Read the model definition and answer for the solid it produces. Units are mm, in the model's axes. Coordinates: 2 decimals unless noted, no trailing zeros. Write each loop counter-clockwise with the first axis right and the second up, starting at its lowest first coordinate (ties: lowest second). Pieces come first, ordered by that corner, then holes.
Item 1: Each of these flat-tipped pins is pushed along its axis until it touches: P1, Ø12.5, axis at x = 12.7, y = -31.24, coming from the +Z side; P2, Ø2, axis at y = 10.5, z = 1, coming from the -X side; P3, Ø1.5, axis at x = -49, z = 2, coming from the -Y side; P4, Ø1, axis at x = 19.5, z = 3, coming from the +Y side. Where does it stop, or does it pass through?
Item 2: Section C-C (z = 1.75) is taken. State how many separate pieces and enclosed holes the cut face has, then the cut area to 3 significant figures.
Item 3: Straight lines are drawn through the part: probe 1 along X at (y, z) = (0.5, 6); probe 2 along X at (y, z) = (-27.5, 4.5); probe 3 along Y at (x, z) = (-12.7, 2.75). For each, find the intervals that lie inside material, in ascending order.
Item 4: Section A-A (x = -31.75) is taken. Give the vertices of the cut face in (y, z) (3 decimals), then the cut area to 3 significant figures.
Item 5: Section B-B (y = 26) is taken. Give the vertices of the cut face in (x, z) (3 decimals).
Item 6: Section D-D (y = -38) is taken. Give the vertices of the cut face in (x, z) (3 decimals), then the cut area to 3 significant figures.
Item 7: Determine the mould class of faces 1 (the face through (0, 49, 3.175)), 2 (the face through (-34.92, 0.14, 3.22)), 3 (the face through (45.486, 14.324, 4.74)), 4 (the face through (20.27, -28.85, 3.22)) for opening direction Y: released by +Y, released by -Y, zero draft, split by the parting line, or undercut.
from build123d import *

# Parameters (mm, degrees)
SKETCH1_R           = 49.5046
BOSS_EXTRUDE1_DEPTH = 3.175
SKETCH2_R           = 47.6885
BOSS_EXTRUDE2_DEPTH = 3.175
SKETCH3_R           = 3.175
SKETCH3_R_2         = 7.9375
CUT_EXTRUDE1_DEPTH  = 7.35
CUT_EXTRUDE2_DEPTH  = 4.175


with BuildPart() as part:
    # Sketch1 → Boss-Extrude1 (new body)
    with BuildSketch(Plane.XY):
        Circle(SKETCH1_R)
    extrude(amount=BOSS_EXTRUDE1_DEPTH)

    # Sketch2 → Boss-Extrude2 (add)
    with BuildSketch(Plane.XY.offset(3.175)):
        Circle(SKETCH2_R)
    extrude(amount=BOSS_EXTRUDE2_DEPTH)

    # Sketch3 → Cut-Extrude1 (cut, through all)
    with BuildSketch(Plane.XY.offset(6.35)):
        with Locations((-31.75, 0)):
            Circle(SKETCH3_R)
        with Locations((31.75, 0)):
            Circle(SKETCH3_R)
        with Locations((-12.7, -31.235352443)):
            Circle(SKETCH3_R_2)
        with Locations((12.7, -31.235352443)):
            Circle(SKETCH3_R_2)
    extrude(amount=-CUT_EXTRUDE1_DEPTH, mode=Mode.SUBTRACT)

    # Sketch4 → Cut-Extrude2 (cut, through all)
    with BuildSketch(Plane.XY.offset(3.175)):
        with BuildLine():
            Line((-50.165, 0), (-47.625, 0))
            ThreePointArc((-47.625, 0), (0, -47.625), (47.625, 0))
            Line((47.625, 0), (50.165, 0))
            ThreePointArc((50.165, 0), (0, -50.165), (-50.165, 0))
        make_face()
    extrude(amount=-CUT_EXTRUDE2_DEPTH, mode=Mode.SUBTRACT)


solid = part.part
Established:
1. P1: passes through
1. P2: stops at x = -48.58
1. P3: stops at y = 0
1. P4: stops at y = 45.71
2. separate pieces: 1
2. enclosed holes: 4
2. area: 6,950 mm2
3. probe 1: x = -47.69 to -34.89, -28.61 to 28.61, 34.89 to 47.69
3. probe 2: x = -38.96 to -19.7, -5.7 to 5.7, 19.7 to 38.96
3. probe 3: y = -45.9 to -39.17, -23.3 to 47.85
4. outline: (-35.583, 3.175) - (-35.498, 3.175) - (-35.498, 0) - (-3.175, 0) - (-3.175, 6.35) - (-35.583, 6.35) - close; (3.175, 0) - (37.982, 0) - (37.982, 3.175) - (35.583, 3.175) - (35.583, 6.35) - (3.175, 6.35) - close
4. area: 419 mm2
5. outline: (-42.127, 0) - (42.127, 0) - (42.127, 3.175) - (39.977, 3.175) - (39.977, 6.35) - (-39.977, 6.35) - (-39.977, 3.175) - (-42.127, 3.175) - close
6. outline: (-28.813, 3.175) - (-28.708, 3.175) - (-28.708, 0) - (-16.853, 0) - (-16.853, 6.35) - (-28.813, 6.35) - close; (-8.547, 0) - (8.547, 0) - (8.547, 6.35) - (-8.547, 6.35) - close; (16.853, 0) - (28.708, 0) - (28.708, 3.175) - (28.813, 3.175) - (28.813, 6.35) - (16.853, 6.35) - close
6. area: 260 mm2
7. face 1: zero draft
7. face 2: undercut
7. face 3: split by the parting line
7. face 4: undercut
